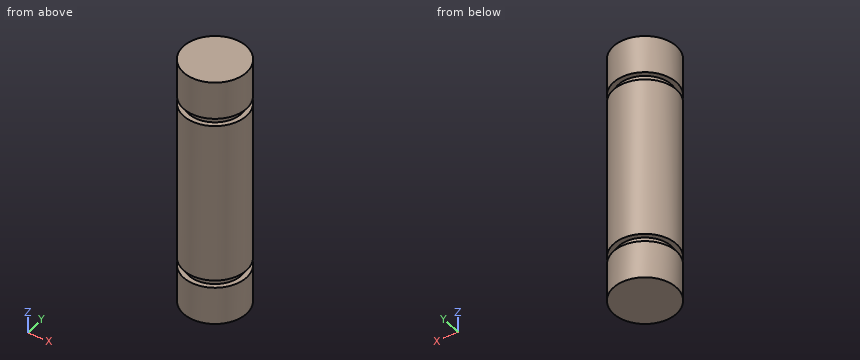
from build123d import *

# Parameters (mm, degrees)
SKETCH1_R           = 3.175
BOSS_EXTRUDE1_DEPTH = 12.7
SKETCH2_W           = 0.508
SKETCH2_H           = 0.762


with BuildPart() as part:
    # Sketch1 → Boss-Extrude1 (new body, symmetric)
    with BuildSketch(Plane.XY):
        Circle(SKETCH1_R)
    extrude(amount=BOSS_EXTRUDE1_DEPTH, both=True)

    # Sketch2 → Cut-Revolve1 (revolve, cut)
    with BuildSketch(Plane(origin=(0, 0, 0), x_dir=(1, 0, 0), z_dir=(0, 1, 0))):
        with Locations((2.921, 8.509)):
            Rectangle(SKETCH2_W, SKETCH2_H)
        with Locations((2.921, -8.509)):
            Rectangle(SKETCH2_W, SKETCH2_H)
    revolve(axis=Axis((0, 0, 12.7), (0, 0, -1)), mode=Mode.SUBTRACT)


solid = part.part
Work out the finished part from the listing and answer in its coordinate system (mm). Round coordinates to 2 decimals unless told otherwise and drop trailing zeros. Write each loop counter-clockwise with the first axis right and the second up, starting at its lowest first coordinate (ties: lowest second). Pieces come first, ordered by that corner, then holes. Notation, with made-up numbers: (0, 33.25) -> (24, 33.25) arc R17 cw to (24, 37.25) -> close; hole circle Ø4 at (16, -39). An arc over 180 degrees is marked (long way). Write each question's results on one line, items separated by ' | '.
Item 1: Find the intervals of material crossed by line 1 along Z through (x, y) = (3, 0); line 2 along X through (y, z) = (-0.5, -3.75); line 3 along X through (y, z) = (-1, 7.75), in increasing order. Write a range as [from, to].
Result set:
line 1: [-12.7, -8.89], [-8.13, 8.13], [8.89, 12.7] | line 2: [-3.14, 3.14] | line 3: [-3.01, 3.01]
Item 2: A cutting plane is placed at A-A, the plane y = -1.5. Determine the outline of the cut face in (x, z), plus the area to 3 significant figures.
Result set:
outline: (-2.8, -12.7) -> (2.8, -12.7) -> (2.8, -8.89) -> (2.21, -8.89) -> (2.21, -8.13) -> (2.8, -8.13) -> (2.8, 8.13) -> (2.21, 8.13) -> (2.21, 8.89) -> (2.8, 8.89) -> (2.8, 12.7) -> (-2.8, 12.7) -> (-2.8, 8.89) -> (-2.21, 8.89) -> (-2.21, 8.13) -> (-2.8, 8.13) -> (-2.8, -8.13) -> (-2.21, -8.13) -> (-2.21, -8.89) -> (-2.8, -8.89) -> close | area: 140 mm^2
Item 3: A flat-ended cylindrical pin translates along its axis: P1, Ø1.5, axis at y = 2.5, z = 3, coming from the -X side. Find the tip coordinate at first contact, or state that the pin passes through.
Result set:
P1: x = -2.65
Item 4: A cutting plane is placed at B-B, the plane x = 1.25. Determine the outline of the cut face in (y, z).
Result set:
outline: (-2.92, -12.7) -> (2.92, -12.7) -> (2.92, -8.89) -> (2.36, -8.89) -> (2.36, -8.13) -> (2.92, -8.13) -> (2.92, 8.13) -> (2.36, 8.13) -> (2.36, 8.89) -> (2.92, 8.89) -> (2.92, 12.7) -> (-2.92, 12.7) -> (-2.92, 8.89) -> (-2.36, 8.89) -> (-2.36, 8.13) -> (-2.92, 8.13) -> (-2.92, -8.13) -> (-2.36, -8.13) -> (-2.36, -8.89) -> (-2.92, -8.89) -> close
Item 5: A cutting plane is placed at C-C, the plane z = -5.5. Determine the outline of the cut face in (x, y) (3 decimals).
Result set:
outline: circle Ø6.35 at (0, 0)
Item 6: A cutting plane is placed at D-D, the plane z = -8.5. Determine the outline of the cut face in (x, y).
Result set:
outline: circle Ø5.33 at (0, 0)
